Input: part model. Units: mm. Frame: model coordinates. Give positions to 0.01 mm unless a question says otherwise; leave off trailing zeros. Order: outer loops, then holes, each group sorted by start corner. A loop starts at its lowest first (then second) coordinate and runs counter-clockwise, first axis right, second up. Notation, with made-up numbers: (69.25, -0.5) - (106.25, -0.5) arc R31 cw to (106.25, 35.5) - close; hole circle Ø6 at (-9.75, 50). An arc over 180 degrees is marked (long way). Answer in a Markdown table with one row per item. Add a question column.
from build123d import *

# Parameters (mm, degrees)
SKETCH1_W           = 1257.3
SKETCH1_H           = 139.7
BOSS_EXTRUDE1_DEPTH = 3.175
SKETCH2_W           = 558.8
SKETCH2_H           = 44.45
CUT_EXTRUDE1_DEPTH  = 4.175
FILLET1_R           = 6.35


with BuildPart() as part:
    # Sketch1 → Boss-Extrude1 (new body)
    with BuildSketch(Plane(origin=(0, 0, 0), x_dir=(1, 0, 0), z_dir=(0, 1, 0))):
        with Locations((628.65, 69.85)):
            Rectangle(SKETCH1_W, SKETCH1_H)
    extrude(amount=BOSS_EXTRUDE1_DEPTH)

    # Sketch2 → Cut-Extrude1 (cut, through all)
    with BuildSketch(Plane(origin=(0, 3.175, 0), x_dir=(1, 0, 0), z_dir=(0, 1, 0))):
        with Locations((628.65, 117.475)):
            Rectangle(SKETCH2_W, SKETCH2_H)
    extrude(amount=-CUT_EXTRUDE1_DEPTH, mode=Mode.SUBTRACT)

    # Fillet1
    fillet1_edges = [part.edges().sort_by_distance(p)[0] for p in [
        (349.25, 1.5875, -95.25),
        (908.05, 1.5875, -95.25),
    ]]
    fillet(fillet1_edges, radius=FILLET1_R)


solid = part.part
Q1. Line query: probe 1 along X at (y, z) = (0.4, -130); probe 2 along Z at (x, y) = (450.5, 1.1). Output: solid intervals per line, ascending.
Q2. Section A-A, the plane y = 1.7. Return loops of the section in (x, z), then the cut area to 3 significant figures.
Q3. Section B-B, the plane x = 558. Return loops of the section in (y, z) (3 decimals).
Computed:
| question | item | result |
|---|---|---|
| 1 | probe 1 | x = 0 to 349.25, 908.05 to 1257.3 |
| 1 | probe 2 | z = -95.25 to 0 |
| 2 | outline | (0, -139.7) - (349.25, -139.7) - (349.25, -101.6) arc R6.35 cw to (355.6, -95.25) - (901.7, -95.25) arc R6.35 cw to (908.05, -101.6) - (908.05, -139.7) - (1257.3, -139.7) - (1257.3, 0) - (0, 0) - close |
| 2 | area | 151,000 mm^2 |
| 3 | outline | (0, -95.25) - (3.175, -95.25) - (3.175, 0) - (0, 0) - close |
